from build123d import *

# Parameters (mm, degrees)
F5_DEPTH = 40


with BuildPart() as f3:
    # F2 (on offset) → F3 section 0
    with BuildSketch(Plane.XY.offset(-30)):
        with BuildLine():
            Line((162.2463304921, -37.5), (162.2463304921, 0))
            Line((162.2463304921, 0), (162.2463304921, 37.5))
            add(Edge.make_bspline(
                [(-72.7536695079, 0), (-29.5158392356, 21.6682380863), (60.1620321507, 64.9393967263), (129.9707958681, 44.834202262), (162.2463304921, 37.5)],
                knots=[0, 0, 0, 0, 0.5444604727, 1, 1, 1, 1], degree=3))
            add(Edge.make_bspline(
                [(-72.7536695079, 0), (-29.5158392356, -21.6682380863), (60.1620321507, -64.9393967263), (129.9707958681, -44.834202262), (162.2463304921, -37.5)],
                knots=[0, 0, 0, 0, 0.5444604727, 1, 1, 1, 1], degree=3))
        make_face()
    # F0 (on Top) → F3 section 1
    with BuildSketch(Plane.XY):
        with BuildLine():
            Line((162.2463304921, -45), (162.2463304921, 0))
            Line((162.2463304921, 0), (162.2463304921, 45))
            add(Edge.make_bspline(
                [(162.2463304921, 45), (150.1698760976, 48.6930710105), (52.7402528222, 64.2426959064), (-14.1104264901, 47.0441984602), (-73.803611279, 8.7933518628), (-87.7536695079, 0)],
                knots=[0, 0, 0, 0, 0.3575982232, 0.6819644283, 1, 1, 1, 1], degree=3))
            add(Edge.make_bspline(
                [(162.2463304921, -45), (150.1698760976, -48.6930710105), (52.7402528222, -64.2426959064), (-14.1104264901, -47.0441984602), (-73.803611279, -8.7933518628), (-87.7536695079, 0)],
                knots=[0, 0, 0, 0, 0.3575982232, 0.6819644283, 1, 1, 1, 1], degree=3))
        make_face()
    loft()

    # F4 (on face) → F5 (cut)
    with BuildSketch(Plane.YZ.offset(162.2463304921)):
        with BuildLine():
            Line((27.5680975042, 0), (-27.5680975042, 0))
            ThreePointArc((-27.5680975042, 0), (0, -20), (27.5680975042, 0))
        make_face()
    extrude(amount=-F5_DEPTH, mode=Mode.SUBTRACT)


solid = f3.part
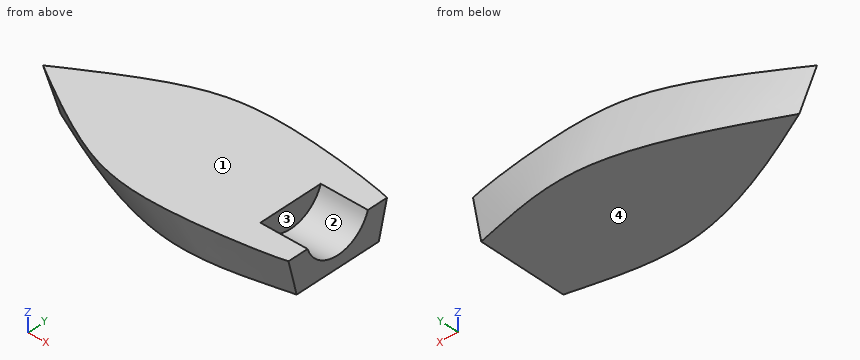
Geometry check sheet. Reference: the model listing, model coordinates, mm. Face numbers are marked on the shaded views. A direction names the side the tool comes from. Round coordinates to 2 decimals unless told otherwise and drop trailing zeros.
Item 1: Gauge pin test, flat ends, axial feed: pin 1 (1.5 mm diameter, centred on x = 50.5, z = -20.5, fed in from -Y); pin 2 (8 mm diameter, centred on y = 7, z = -7.5, fed in from +X); pin 3 (1 mm diameter, centred on x = 115, z = -3, fed in from +Y). Record the tip position at first contact, or that the pin passes through.
Item 2: Thickness scan on line 1 (Y direction, x = 124, z = -4); line 2 (X direction, y = 19.5, z = -28); line 3 (Y direction, x = 104, z = -20.5). Record the ranges inside material, lowest first.
Item 3: Mould release check, pull along Y, two halves, no side actions. Record for the marked faces 1 and 2: pulls with the +Y half, pulls with the -Y half, needs draft (parallel to the pull), parting line crosses it, or undercut.
Item 4: Access from +Z, -Z, +X, -X, +Y, -Y to the whole of each face (thin tool, end or side, straight path). Record for the marked faces 3 and 4.
Answer sheet:
1. pin 1: stops at y = -51.9
1. pin 2: stops at x = 122.25
1. pin 3: stops at y = 52.79
2. line 1: y = -51.24 to -25.92, 25.92 to 51.24
2. line 2: x = -34.12 to 162.25
2. line 3: y = -50.96 to 50.96
3. face 1: needs draft
3. face 2: undercut
4. face 3: +Z, +X
4. face 4: -Z, +X, -X, +Y, -Y
